Input: part model. Units: mm. Frame: model coordinates. A direction names the side the tool comes from. Round coordinates to 2 decimals unless told otherwise and drop trailing zeros. Return JSON: item names as keys, results as strings. Group by question number.
1) Access query for faces 4 (the face through (5.3, 0.1, -0.1)), 5 (the face through (13.1, -5.97, 0.05)). Directions: +Z, -Z, +X, -X, +Y, -Y. A direction counts if a zero-diameter tool reaches every point of the face in a straight line with its end or side. Return the directions, or none.
2) Contact query for flat-ended pins moving along their axis: P1, Ø3, axis at x = 3, y = -6, coming from the -Z side; P2, Ø1.5, axis at x = 9.5, z = -1, coming from the -Y side. Output: stop coordinate, or through.
3) Material intervals for line 1 (X direction, y = -3.25, z = 0); line 2 (Z direction, x = 10.75, y = -1.25); line 3 (Z direction, x = 6.75, y = -0.5), sorted ascending. Write a range as from..to.
4) Mould query, pull axis Z, two halves, no side actions, for faces 1 (the face through (14.83, -5.4, -0.29)), 2 (the face through (11.212, -4.64, -0.901)), 3 (the face through (14.3, -2.935, 3.1)). Classes: +Z half, -Z half, draft (parallel to the pull), parting line (faces both ways), or undercut.
from build123d import *

# Parameters (mm, degrees)
SKETCH117_R           = 3
CUT_EXTRUDE4_DEPTH    = 3
SKETCH122_R           = 6.539767279
BOSS_EXTRUDE1_DEPTH   = 5
M2X0_4_TAPPED_HOLE1_D = 1.6
SKETCH125_R           = 3
CUT_EXTRUDE5_DEPTH    = 7


with BuildPart() as part:
    # Sketch9 → Revolve1 (revolve)
    with BuildSketch(Plane.XY):
        with BuildLine():
            Line((-4.703089141, -2.935363462), (8.296910859, -2.935363462))
            Line((8.296910859, -2.935363462), (8.296910859, 1.564636538))
            Line((8.296910859, 1.564636538), (-4.703089141, 1.564636538))
            add(Edge.make_bspline(
                [(-4.703089141, 1.564636538), (8.296910859, -1.435363462), (-4.703089141, -2.935363462)],
                knots=[0, 0, 0, 1, 1, 1], degree=2))
        make_face()
    revolve(axis=Axis((8.296910859, -2.935363462, 0), (0, 1, 0)))

    # Sketch117 → Cut-Extrude4 (cut)
    with BuildSketch(Plane(origin=(0, 1.564636538, 0), x_dir=(1, 0, 0), z_dir=(0, 1, 0))):
        with Locations((8.29691086, 0)):
            Circle(SKETCH117_R)
    extrude(amount=-CUT_EXTRUDE4_DEPTH, mode=Mode.SUBTRACT)

    # Sketch122 → Boss-Extrude1 (add)
    with BuildSketch(Plane(origin=(0, -2.935363462, 0), x_dir=(-1, 0, 0), z_dir=(0, -1, 0))):
        with Locations((-8.29691086, 0)):
            Circle(SKETCH122_R)
    extrude(amount=BOSS_EXTRUDE1_DEPTH)

    # M2x0.4 Tapped Hole1 (through all)
    with Locations(Plane(origin=(1.815385484, -5.431649491, -0.870852953), x_dir=(0.133162682, 0, -0.991094193), z_dir=(-0.991094193, 0, -0.133162682))):
        with Locations((0, 0)):
            Hole(M2X0_4_TAPPED_HOLE1_D / 2)

    # Sketch125 → Cut-Extrude5 (cut)
    with BuildSketch(Plane(origin=(0, -1.435363462, 0), x_dir=(1, 0, 0), z_dir=(0, 1, 0))):
        with Locations((8.350281981, 0)):
            Circle(SKETCH125_R)
    extrude(amount=-CUT_EXTRUDE5_DEPTH, mode=Mode.SUBTRACT)


solid = part.part
Returned:
{
 "1": {"face 4": "+Y", "face 5": "none"},
 "2": {"P1": "stops at z = -5.32", "P2": "passes through"},
 "3": {"line 1": "x = 1.76..5.35, 11.35..14.84", "line 2": "z = -6.07..-1.73, 1.73..6.07", "line 3": "z = -6.7..-2.57, 2.57..6.7"},
 "4": {"face 1": "parting line", "face 2": "undercut", "face 3": "draft"}
}
